Work out the finished part from the listing and answer in its coordinate system (mm). A direction names the side the tool comes from. Give positions to 0.01 mm unless a question says otherwise; leave off trailing zeros. Order: outer loops, then holes, each group sorted by start corner. A loop starts at its lowest first (then second) coordinate and runs counter-clockwise, first axis right, second up. Notation, with made-up numbers: (59, 29) - (107, 29) arc R28 ccw to (107, 56) - close; hole circle Ø3 at (-12, 33). An arc over 180 degrees is marked (long way). Put each result on its own line as item: value.
```python
from build123d import *

# Parameters (mm, degrees)
SKETCH_2_R               = 1.5
CUT_EXTRUDE_1_DEPTH      = 6
PATTERN_CIRCULAR_1_COUNT = 6
SKETCH_3_R               = 1.5
CUT_EXTRUDE_2_DEPTH      = 81.725212914
PATTERN_CIRCULAR_2_COUNT = 6
SKETCH_4_R               = 49.8
CUT_EXTRUDE_3_DEPTH      = 5


with BuildPart() as part:
    # 草图1 → 旋转1 (revolve)
    with BuildSketch(Plane.XY, mode=Mode.PRIVATE) as revolve_1_sk:
        Polygon((0, 41.5), (0, 50), (4.32, 50), (4.32, 46), (8.64, 46), (8.64, 50), (12.96, 50), (12.96, 46), (17.28, 46), (17.28, 50), (21.6, 50), (21.6, 55), (27.6, 55), (27.6, 41.5), align=None)
    revolve(revolve_1_sk.sketch.rotate(Axis((27.6, 0, 0), (1, 0, 0)), 180), axis=Axis((27.6, 0, 0), (1, 0, 0)))

    # 草图2 → 切除-拉伸1 (cut)
    with BuildSketch(Plane.ZY):
        with Locations(Location((0, 44, 0), (0, 0, 270))):
            Circle(SKETCH_2_R)
    cut_extrude_1 = extrude(amount=-CUT_EXTRUDE_1_DEPTH, mode=Mode.SUBTRACT)

    # 阵列(圆周)1: 切除-拉伸1 ×6 about axis
    pattern_circular_1_axis = Axis((0, 0, 0), (1, 0, 0))
    for i in range(1, PATTERN_CIRCULAR_1_COUNT):
        add(cut_extrude_1.rotate(pattern_circular_1_axis, i * 360 / PATTERN_CIRCULAR_1_COUNT), mode=Mode.SUBTRACT)

    # 草图3 → 切除-拉伸2 (cut, symmetric)
    with BuildSketch(Plane.ZY.offset(-21.6)):
        with Locations((0, 52.5)):
            Circle(SKETCH_3_R)
    cut_extrude_2 = extrude(amount=CUT_EXTRUDE_2_DEPTH, both=True, mode=Mode.SUBTRACT)

    # 阵列(圆周)2: 切除-拉伸2 ×6 about axis
    pattern_circular_2_axis = Axis((0, 0, 0), (1, 0, 0))
    for i in range(1, PATTERN_CIRCULAR_2_COUNT):
        add(cut_extrude_2.rotate(pattern_circular_2_axis, i * 360 / PATTERN_CIRCULAR_2_COUNT), mode=Mode.SUBTRACT)

    # 草图4 → 切除-拉伸3 (cut)
    with BuildSketch(Plane(origin=(27.6, 0, 0), x_dir=(0, 0, -1), z_dir=(1, 0, 0))):
        with Locations(Location((0, 0, 0), (0, 0, 90))):
            Circle(SKETCH_4_R)
    extrude(amount=-CUT_EXTRUDE_3_DEPTH, mode=Mode.SUBTRACT)


solid = part.part
```
(1) Section D-D, the plane y = 52.5 is taken. Write down the section's boundary in (x, z), then the cut area to 3 significant figures.
Geometry check:
outline: (21.6, -16.39) - (27.6, -16.39) - (27.6, -1.5) - (21.6, -1.5) - close; (21.6, 1.5) - (27.6, 1.5) - (27.6, 16.39) - (21.6, 16.39) - close
area: 179 mm²
(2) Straight lines are drawn through the part: line 1 (Z direction, x = 4.55, y = 22); line 2 (Y direction, x = 3.25, z = -3); line 3 (Z direction, x = 22.5, y = -29.5). For each, find the intervals that lie inside material, in ascending order.
Geometry check:
line 1: z = -40.4 to -39.61, -36.61 to -35.19, 35.19 to 36.61, 39.61 to 40.4
line 2: y = -49.91 to -41.39, 41.39 to 49.91
line 3: z = -46.42 to -29.19, 29.19 to 46.42
(3) Given pin 1 (4 mm diameter, centred on y = -52.5, z = 0, fed in from +X); pin 2 (1.5 mm diameter, centred on y = 22, z = -37.5, fed in from -X); pin 3 (4 mm diameter, centred on x = 24, y = 40, fed in from -Z); pin 4 (6 mm diameter, centred on x = 16, y = 22, fed in from +Z), each flat-ended and moving along its own axis, determine where each tip first touches the part or whether it passes through.
Geometry check:
pin 1: stops at x = 27.6
pin 2: stops at x = 6
pin 3: stops at z = -39.76
pin 4: stops at z = 46.13
(4) A tool of negligible diameter and unlimited length cuts with its end or side. For faces 5 (the face through (22.6, -11, 41)), 6 (the face through (2.958, 22.806, 36.84)), 7 (the face through (8.64, 22, 41)), from which of +Z, -Z, +X, -X, +Y, -Y can it reach the whole face along a straight path? Write none if from no direction.
Geometry check:
face 5: +X
face 6: -X
face 7: none
(5) Determine the mould class of faces 1 (the face through (4.32, -22, 41)), 2 (the face through (6.51, 5.99, -45.61)), 3 (the face through (6, -22, 38)), 4 (the face through (2.96, -21.8, 39.59)) for opening direction Y: pulls with the +Y half, pulls with the -Y half, needs draft (parallel to the pull), parting line crosses it, or undercut.
Geometry check:
face 1: needs draft
face 2: parting line crosses it
face 3: undercut
face 4: undercut
(6) Section C-C, the plane x = 24.25 is taken. Write down the section's boundary in (y, z).
Geometry check:
outline: circle Ø110 at (0, 0); hole circle Ø3 at (-52.5, 0); hole circle Ø99.6 at (0, 0); hole circle Ø3 at (-26.25, -45.47); hole circle Ø3 at (-26.25, 45.47); hole circle Ø3 at (26.25, -45.47); hole circle Ø3 at (26.25, 45.47); hole circle Ø3 at (52.5, 0)
